Geometry check sheet. Reference: the model listing, model coordinates, mm. Face numbers are marked on the shaded views. A direction names the side the tool comes from. Give positions to 0.01 mm unless a question says otherwise; leave off trailing zeros. Order: outer loops, then holes, each group sorted by start corner. A loop starts at its lowest first (then second) coordinate and runs counter-clockwise, first axis right, second up.
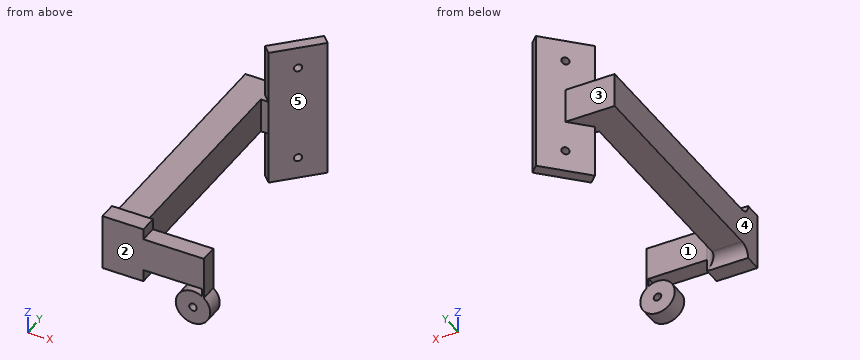
```python
from build123d import *

# Parameters (mm, degrees)
BOSS_EXTRUDE2_DEPTH      = 65
CUT_EXTRUDE1_DEPTH       = 82.266390279
CUT_EXTRUDE1_DEPTH_BACK  = 82.266390279
SKETCH4_R                = 1.75
BOSS_EXTRUDE3_DEPTH      = 8
BOSS_EXTRUDE3_DEPTH_BACK = 8
BOSS_EXTRUDE3_START      = -32.5
SKETCH9_W                = 14
SKETCH9_H                = 16
BOSS_EXTRUDE4_DEPTH      = 100
SKETCH10_R               = 1.75
BOSS_EXTRUDE5_DEPTH      = 8
FILLET4_R                = 5


with BuildPart() as part:
    # Sketch3 → Boss-Extrude2 (new body)
    with BuildSketch(Plane.XY):
        Polygon((-3.535533906, 33.535533906), (0, 30), (17.67766953, 47.67766953), (14.142135624, 51.213203436), align=None)
    extrude(amount=-BOSS_EXTRUDE2_DEPTH)

    # Sketch4 → Cut-Extrude1 (cut, two sides: drawn at the far end of the back side and taken through both)
    with BuildSketch(Plane(origin=(-18.535533906, 18.535533906, 0), x_dir=(0, 0, 1), z_dir=(-0.7071067811865477, 0.7071067811865475, 0)).offset(-CUT_EXTRUDE1_DEPTH_BACK)):
        with Locations(Location((-10, 33.713203436, 0), (0, 0, 270))):
            Circle(SKETCH4_R)
        with Locations(Location((-55, 33.713203436, 0), (0, 0, 270))):
            Circle(SKETCH4_R)
    extrude(amount=CUT_EXTRUDE1_DEPTH + CUT_EXTRUDE1_DEPTH_BACK, mode=Mode.SUBTRACT)

    # Sketch8 → Boss-Extrude3 (add, two sides: drawn at the far end of the back side and taken through both)
    with BuildSketch(Plane(origin=(0, 0, -65), x_dir=(-1, 0, 0), z_dir=(0, 0, -1)).offset(BOSS_EXTRUDE3_START - BOSS_EXTRUDE3_DEPTH_BACK)):
        Polygon((-5.303300859, 42.374368671), (17.535533906, 42.374368671), (17.535533906, 30), (0, 30), (3.535533906, 33.535533906), align=None)
    extrude(amount=BOSS_EXTRUDE3_DEPTH + BOSS_EXTRUDE3_DEPTH_BACK)

    # Sketch9 → Boss-Extrude4 (add)
    with BuildSketch(Plane.XZ.offset(-30)):
        with Locations((-10.535533906, -32.5)):
            Rectangle(SKETCH9_W, SKETCH9_H)
    extrude(amount=BOSS_EXTRUDE4_DEPTH)

    # Sketch10 → Boss-Extrude5 (add)
    with BuildSketch(Plane.XZ.offset(70)):
        with BuildLine():
            Line((29.465894629, -44.217395538), (29.465894629, -24.5))
            Line((29.465894629, -24.5), (1.464466094, -24.5))
            Line((1.464466094, -24.5), (1.464466094, -19.5))
            Line((1.464466094, -19.5), (-17.535533906, -19.5))
            Line((-17.535533906, -19.5), (-17.535533906, -45.5))
            Line((-17.535533906, -45.5), (1.464466094, -45.5))
            Line((1.464466094, -45.5), (1.464466094, -39.889528684))
            Line((1.464466094, -39.889528684), (28.589308321, -39.889528684))
            Line((28.589308321, -39.889528684), (28.589308321, -43.606924222))
            ThreePointArc((28.589308321, -43.606924222), (19.893987133, -57.027274483), (29.465894629, -44.217395538))
        make_face()
        with Locations(Location((24.465894629, -50.462393537, 0), (0, 0, 270))):
            Circle(SKETCH10_R, mode=Mode.SUBTRACT)
    extrude(amount=BOSS_EXTRUDE5_DEPTH)

    # Fillet4
    fillet4_edges = [part.edges().sort_by_distance(p)[0] for p in [
        (-10.535533906, -70, -40.5),
        (-10.535533906, -70, -24.5),
        (-3.535533906, -70, -32.5),
    ]]
    fillet(fillet4_edges, radius=FILLET4_R - 0.0001)  # a hair under: the kernel refuses the full size


solid = part.part
```
Q1. Cross-section at B-B, the plane z = -6.5. Record the boundary of the cut face in (x, y).
Q2. Access from +Z, -Z, +X, -X, +Y, -Y to the whole of each face (thin tool, end or side, straight path). Record for the marked faces 1 and 2.
Q3. Release check for a two-part mould opening along Y. For the marked faces 3, 4 and 5 record: pulls with the +Y half, pulls with the -Y half, needs draft (parallel to the pull), parting line crosses it, or undercut.
Q4. Cross-section at C-C, the plane y = 36. Record the boundary of the cut face in (x, z).
Q5. Gauge pin test, flat ends, axial feed: P1, Ø3, axis at x = 11, z = -9, coming from the +Y side; P2, Ø4, axis at y = -72, z = -36.5, coming from the +X side; P3, Ø8, axis at y = 6, z = -22, coming from the -X side; P4, Ø8, axis at y = 3, z = -29, coming from the +X side. Record the tip position at first contact, or that the pin passes through.
Q6. Cross-section at D-D, the plane y = -45. Record the boundary of the cut face in (x, z), and give its area (3 significant figures).
Q7. Thickness scan on L1, parallel to Z at x = -3, y = 35; L2, parallel to Y at x = 21, z = -44; L3, parallel to X at y = -11.5, z = -34.5. Record the ranges inside material, lowest first.
Answers follow:
1. outline: (-3.54, 33.54) - (0, 30) - (17.68, 47.68) - (14.14, 51.21) - close
2. face 1: +Z, -Z, +X
2. face 2: +Z, -Z, +X, -X, -Y
3. face 3: pulls with the +Y half
3. face 4: needs draft
3. face 5: undercut
4. outline: (-17.54, -40.5) - (-1.07, -40.5) - (-1.07, -65) - (6, -65) - (6, 0) - (-1.07, 0) - (-1.07, -24.5) - (-17.54, -24.5) - close
5. P1: stops at y = 49.57
5. P2: stops at x = 29.47
5. P3: stops at x = -17.54
5. P4: stops at x = -3.54
6. outline: (-17.54, -40.5) - (-3.54, -40.5) - (-3.54, -24.5) - (-17.54, -24.5) - close
6. area: 224 mm2
7. L1: z = -40.5 to -24.5
7. L2: y = -78 to -70
7. L3: x = -17.54 to -3.54
